Study the drawing (mm; zero at the part's minimum x, y, z) and answer. A direction names the side the tool comes from. Coordinates: 2 decimals unless noted, no trailing zeros. Order: outer loops, then holes, each group sorted by start corner. A loop starts at its lowest first (then second) coordinate and runs counter-clockwise, first axis right, second up. Notation, with made-up numbers: M -3.5,-21.5 L 1.5,-21.5 A33 cw 1.5,11.5 Z; hole C 13.5,78.25 d2. An arc over 180 degrees is marked long. Put each result on its own line as item: value.
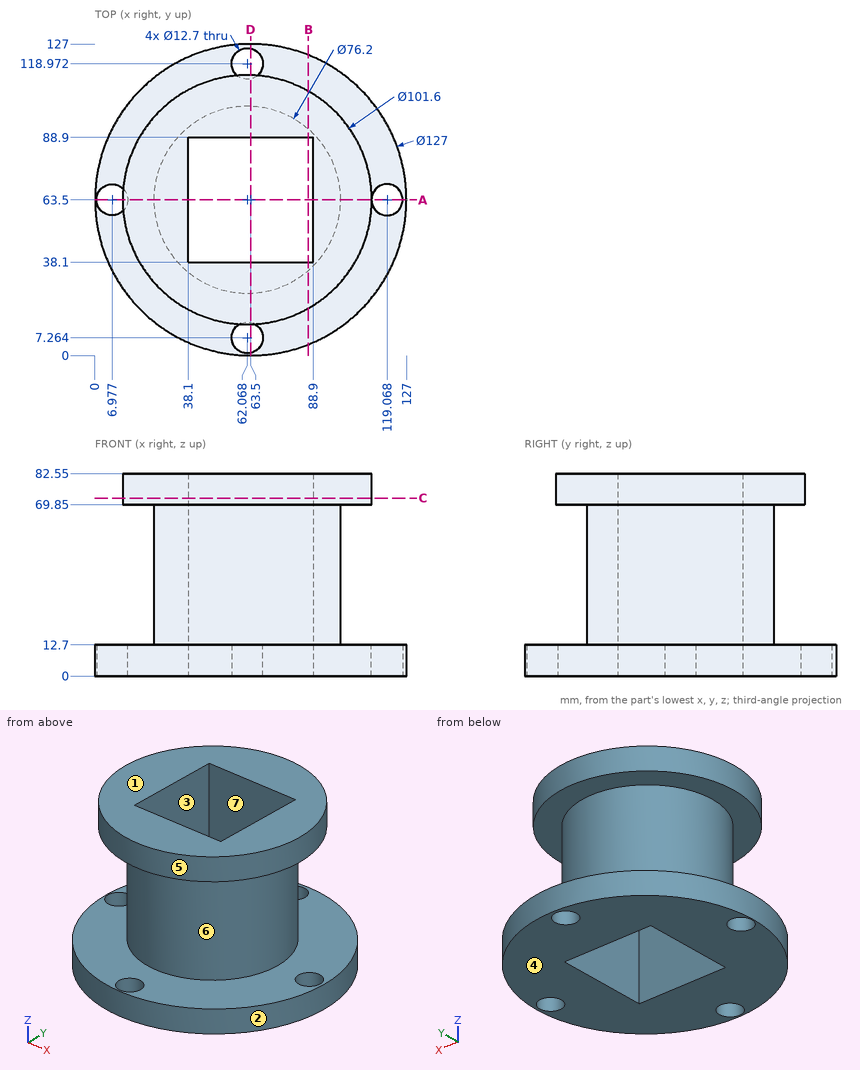
Q1. Find section B-B on x = 87. Write down the section's boundary in (y, z).
Answers below:
outline: M 4.51,0 L 38.1,0 L 38.1,82.55 L 19.24,82.55 L 19.24,69.85 L 34.69,69.85 L 34.69,12.7 L 4.51,12.7 Z; M 88.9,0 L 122.49,0 L 122.49,12.7 L 92.31,12.7 L 92.31,69.85 L 107.76,69.85 L 107.76,82.55 L 88.9,82.55 Z
Q2. Given pin 1 (2 mm diameter, centred on y = 74.5, z = 33.5, fed in from +X); pin 2 (1 mm diameter, centred on x = 75.5, z = 50, fed in from -Y); pin 3 (15 mm diameter, centred on x = 66.5, z = 21.5, fed in from +Y), each flat-ended and moving along its own axis, determine where each tip first touches the part or whether it passes through.
Answers below:
pin 1: stops at x = 98.83
pin 2: stops at y = 27.66
pin 3: stops at y = 101.6
Q3. Consider line 1 along Z through (x, y) = (18, 80.5); line 2 along X through (y, z) = (66.5, 9) (1 decimal); line 3 along Z through (x, y) = (28, 103.5). Determine where each line is inside the solid, lowest interval first.
Answers below:
line 1: z = 0 to 12.7, 69.85 to 82.55
line 2: x = 0.1 to 1.4, 12.6 to 38.1, 88.9 to 113.5, 124.7 to 126.9
line 3: z = 0 to 12.7
Q4. A tool of negligible diameter and unlimited length cuts with its end or side. For the marked faces 4, 5, 6 and 7, from which of +Z, -Z, +X, -X, +Y, -Y can it reach the whole face along a straight path? Write none if from no direction.
Answers below:
face 4: -Z, +X, -X, +Y, -Y
face 5: +Z
face 6: none
face 7: +Z, -Z
Q5. Find section C-C on z = 72.5. Write down the section's boundary in (x, y).
Answers below:
outline: C 62.07,63.5 d101.6; hole M 38.1,38.1 L 88.9,38.1 L 88.9,88.9 L 38.1,88.9 Z
Q6. Find section A-A on y = 63.5. Write down the section's boundary in (x, z).
Answers below:
outline: M 0,0 L 0.63,0 L 0.63,12.7 L 0,12.7 Z; M 11.27,69.85 L 23.97,69.85 L 23.97,12.7 L 13.33,12.7 L 13.33,0 L 38.1,0 L 38.1,82.55 L 11.27,82.55 Z; M 88.9,0 L 112.72,0 L 112.72,12.7 L 100.17,12.7 L 100.17,69.85 L 112.87,69.85 L 112.87,82.55 L 88.9,82.55 Z; M 125.42,0 L 127,0 L 127,12.7 L 125.42,12.7 Z
Q7. Find section D-D on x = 63.5. Write down the section's boundary in (y, z), plus the area to 3 significant figures.
Answers below:
outline: M 0,0 L 1.08,0 L 1.08,12.7 L 0,12.7 Z; M 12.72,69.85 L 25.43,69.85 L 25.43,12.7 L 13.45,12.7 L 13.45,0 L 38.1,0 L 38.1,82.55 L 12.72,82.55 Z; M 88.9,0 L 112.79,0 L 112.79,12.7 L 101.57,12.7 L 101.57,69.85 L 114.28,69.85 L 114.28,82.55 L 88.9,82.55 Z; M 125.16,0 L 127,0 L 127,12.7 L 125.16,12.7 Z
area: 2,750 mm^2
Q8. For a pull along X with two mould halves and no side action, classify the marked faces 1, 2 and 3 as +X half, -X half, draft (parallel to the pull), parting line (faces both ways), or undercut.
Answers below:
face 1: draft
face 2: parting line
face 3: undercut
